from build123d import *

# Parameters (mm, degrees)
F0_W            = 130
F0_H            = 200
F1_DEPTH        = 12
F3_D            = 5.5
F3_CBORE_D      = 9.75
F3_CBORE_DEPTH  = 5
F5_DEPTH        = 25
F7_DEPTH        = 6
F9_DEPTH        = 2
F11_D           = 5.1
F11_CBORE_D     = 11
F11_CBORE_DEPTH = 6
F13_D           = 5
F13_CBORE_D     = 10
F13_CBORE_DEPTH = 6
F15_D           = 4.1


with BuildPart() as f1:
    # F0 (on Top) → F1 (new body)
    with BuildSketch(Plane.XY):
        Rectangle(F0_W, F0_H)
    extrude(amount=F1_DEPTH)

    # F3 (through all)
    with Locations(Plane.XY.offset(12)):
        with Locations((-50, -90), (0, -90), (50, -90), (-50, 10), (-50, 35), (50, 10), (50, 35), (-50, 85), (50, 85), (0, -15)):
            CounterBoreHole(F3_D / 2, F3_CBORE_D / 2, F3_CBORE_DEPTH)

    # F4 (on face) → F5 (cut)
    with BuildSketch(Plane.XY.offset(12)):
        with BuildLine():
            ThreePointArc((-19.5, 37), (-22, 39.5), (-24.5, 37))
            Line((-24.5, 37), (-24.5, 31))
            ThreePointArc((-24.5, 31), (-22, 28.5), (-19.5, 31))
            Line((-19.5, 31), (-19.5, 37))
        make_face()
        with BuildLine():
            ThreePointArc((24.5, 37), (22, 39.5), (19.5, 37))
            Line((19.5, 37), (19.5, 31))
            ThreePointArc((19.5, 31), (22, 28.5), (24.5, 31))
            Line((24.5, 31), (24.5, 37))
        make_face()
    extrude(amount=-F5_DEPTH, mode=Mode.SUBTRACT)

    # F6 (on face) → F7 (cut)
    with BuildSketch(Plane(origin=(0, 0, 0), x_dir=(1, 0, 0), z_dir=(0, 0, -1))):
        with BuildLine():
            ThreePointArc((17, -37), (22, -42), (27, -37))
            Line((27, -37), (27, -31))
            ThreePointArc((27, -31), (22, -26), (17, -31))
            Line((17, -31), (17, -37))
        make_face()
        with BuildLine():
            Line((24.5, -31), (24.5, -37))
            ThreePointArc((24.5, -37), (22, -39.5), (19.5, -37))
            Line((19.5, -37), (19.5, -31))
            ThreePointArc((19.5, -31), (22, -28.5), (24.5, -31))
        make_face(mode=Mode.SUBTRACT)
        with BuildLine():
            Line((-27, -31), (-27, -37))
            ThreePointArc((-27, -37), (-22, -42), (-17, -37))
            Line((-17, -37), (-17, -31))
            ThreePointArc((-17, -31), (-22, -26), (-27, -31))
        make_face()
        with BuildLine():
            Line((-19.5, -31), (-19.5, -37))
            ThreePointArc((-19.5, -37), (-22, -39.5), (-24.5, -37))
            Line((-24.5, -37), (-24.5, -31))
            ThreePointArc((-24.5, -31), (-22, -28.5), (-19.5, -31))
        make_face(mode=Mode.SUBTRACT)
    extrude(amount=-F7_DEPTH, mode=Mode.SUBTRACT)

    # F8 (on face) → F9 (cut)
    with BuildSketch(Plane.XY.offset(12)):
        with BuildLine():
            Line((-18.3303027798, -64), (18.3303027798, -64))
            ThreePointArc((18.3303027798, -64), (25, -47), (18.3303027798, -30))
            Line((18.3303027798, -30), (-18.3303027798, -30))
            ThreePointArc((-18.3303027798, -30), (-25, -47), (-18.3303027798, -64))
        make_face()
    extrude(amount=-F9_DEPTH, mode=Mode.SUBTRACT)

    # F11 (through all)
    with Locations(Plane(origin=(0, 0, 0), x_dir=(1, 0, 0), z_dir=(0, 0, -1))):
        with Locations((20, 47), (-20, 47)):
            CounterBoreHole(F11_D / 2, F11_CBORE_D / 2, F11_CBORE_DEPTH)

    # F13 (through all)
    with Locations(Plane(origin=(0, 0, 0), x_dir=(1, 0, 0), z_dir=(0, 0, -1))):
        with Locations((57.5, 57.5), (57.5, 37.5), (-57.5, 57.5), (-57.5, 37.5), (57.5, 25), (57.5, 5), (-57.5, 25), (-57.5, 5), (-42.5, 70), (42.5, 70)):
            CounterBoreHole(F13_D / 2, F13_CBORE_D / 2, F13_CBORE_DEPTH)

    # F15 (through all)
    with Locations(Plane.XY.offset(12)):
        with Locations((22, 1), (-22, 1)):
            Hole(F15_D / 2)


solid = f1.part
Can you work these out from the model? Positions are in its coordinate system, mm. A direction names the side the tool comes from. Coordinates: 2 decimals unless noted, no trailing zeros. Write each loop counter-clockwise with the first axis right and the second up, starting at its lowest first coordinate (ties: lowest second). Pieces come first, ordered by that corner, then holes. Notation, with made-up numbers: (-29, 18.5) -> (26, 18.5) arc R14 ccw to (26, 32.5) -> close; hole circle Ø7 at (-21.75, 16). An arc over 180 degrees is marked (long way). Write each question's results on one line, items separated by ' | '. Start each with the question number.
Q1. If I drill on probe 1 along X at (y, z) = (-86, 11); probe 2 along X at (y, z) = (-25, 4.1); probe 3 along Y at (x, z) = (-50, 2.5), over which ranges is the centre line in solid material (lowest first)?
Q2. On a 3-axis mill with a long thin cutter (end or side, diameter ignored), from which of +Z, -Z, +X, -X, +Y, -Y can I reach the whole of each face in a straight line? I mean faces 1 (the face through (-21.9, 39.5, 9)), 2 (the face through (0, -47, 10)), 3 (the face through (55, -4, 6)). Say none if no direction works.
Q3. We'd pull the mould along Y, two halves only. Please class faces 4 (the face through (-65, -1, 6)), 5 (the face through (25, -47, 11)): +Y half, -Y half, draft (parallel to the pull), parting line (faces both ways), or undercut.
Q4. Imagine slicing it at D-D (y = 85). Write out the boundary of the cut face in (x, z) (3 decimals).
Q5. Imagine slicing it at C-C (y = -47). Write out the boundary of the cut face in (x, z), then the cut area to 3 significant figures.
Q6. Imagine slicing it at A-A (y = -15). Write out the boundary of the cut face in (x, z) (3 decimals), then the cut area to 3 significant figures.
Q7. I'm going to push flat-ended pins straight in: pin 1 (3.5 mm diameter, centred on x = -20, y = -49, fed in from -Z); pin 2 (4.5 mm diameter, centred on x = -57.5, y = -25, fed in from +Z); pin 3 (5 mm diameter, centred on x = -51, y = 33, fed in from +Z). Where does each tip first touch, or does it pass through?
Q8. Imagine slicing it at B-B (x = -43). Write out the boundary of the cut face in (y, z).
Taken from the geometry:
1) probe 1: x = -65 to -52.79, -47.21 to -2.79, 2.79 to 47.21, 52.79 to 65 | probe 2: x = -65 to -62.5, -52.5 to 52.5, 62.5 to 65 | probe 3: y = -100 to -92.75, -87.25 to 7.25, 12.75 to 32.25, 37.75 to 82.25, 87.75 to 100
2) face 1: +Z, -Z | face 2: +Z | face 3: -Z
3) face 4: draft | face 5: undercut
4) outline: (-65, 0) -> (-52.75, 0) -> (-52.75, 7) -> (-54.875, 7) -> (-54.875, 12) -> (-65, 12) -> close; (-47.25, 0) -> (47.25, 0) -> (47.25, 7) -> (45.125, 7) -> (45.125, 12) -> (-45.125, 12) -> (-45.125, 7) -> (-47.25, 7) -> close; (52.75, 0) -> (65, 0) -> (65, 12) -> (54.875, 12) -> (54.875, 7) -> (52.75, 7) -> close
5) outline: (-65, 0) -> (-25.5, 0) -> (-25.5, 6) -> (-22.55, 6) -> (-22.55, 10) -> (-25, 10) -> (-25, 12) -> (-65, 12) -> close; (-17.45, 6) -> (-14.5, 6) -> (-14.5, 0) -> (14.5, 0) -> (14.5, 6) -> (17.45, 6) -> (17.45, 10) -> (-17.45, 10) -> close; (22.55, 6) -> (25.5, 6) -> (25.5, 0) -> (65, 0) -> (65, 12) -> (25, 12) -> (25, 10) -> (22.55, 10) -> close | area: 1,290 mm^2
6) outline: (-65, 0) -> (-2.75, 0) -> (-2.75, 7) -> (-4.875, 7) -> (-4.875, 12) -> (-65, 12) -> close; (2.75, 0) -> (65, 0) -> (65, 12) -> (4.875, 12) -> (4.875, 7) -> (2.75, 7) -> close | area: 1,470 mm^2
7) pin 1: stops at z = 6 | pin 2: passes through | pin 3: stops at z = 7
8) outline: (-100, 0) -> (-74.97, 0) -> (-74.97, 6) -> (-72.45, 6) -> (-72.45, 12) -> (-100, 12) -> close; (-67.55, 6) -> (-65.03, 6) -> (-65.03, 0) -> (100, 0) -> (100, 12) -> (-67.55, 12) -> close
